The listing builds one solid part. Answer for the finished solid, in the listing's coordinates (mm). A direction names the side the tool comes from. Give positions to 0.01 mm unless a question says otherwise; leave off trailing zeros. Write each loop counter-clockwise with the first axis right and the second up, starting at its lowest first coordinate (ties: lowest second). Pieces come first, ordered by that corner, then holes. Notation, with made-up numbers: M 12,38.5 L 53,38.5 A19 cw 53,57.5 Z; hole C -17.5,-26.5 d11. An arc over 180 degrees is marked long. Return JSON: item names as keys, results as strings.
from build123d import *

# Parameters (mm, degrees)
POCKET002_DEPTH      = 20.001
POCKET002_DEPTH_BACK = -20.001
POCKET003_DEPTH      = 5
SKETCH004_R          = 5.2
POCKET004_DEPTH      = 26.045604
POCKET004_DEPTH_BACK = -21.981715
SKETCH007_R          = 15.2
SKETCH_R             = 20
SKETCH_R_2           = 15.3
PAD_DEPTH            = 9
SKETCH001_R          = 1.7
POCKET_DEPTH         = 134.561028
SKETCH002_R          = 2.95
POCKET001_DEPTH      = 2.5
SKETCH006_R          = 5.2
POCKET005_DEPTH      = 14.143136
POLARPATTERN_COUNT   = 3


with BuildPart() as body001:
    # Cone → Cone (revolve)
    with BuildSketch(Plane(origin=(0, 0, 9), x_dir=(1, 0, 0), z_dir=(0, -1, 0))):
        Polygon((0, 0), (20, 0), (0, 50), align=None)
    revolve(axis=Axis((0, 0, 9), (0, 0, 1)))

    # Sketch003 → Pocket002 (cut, two sides)
    with BuildSketch(Plane.YZ) as pocket002_sk:
        Polygon((22.25, 62.25), (-22.25, 17.75), (-27.75, 17.75), (-27.75, 67.75), (22.25, 67.75), align=None)
        Polygon((30.213203, 9), (-4.786797, 9), (-4.786797, 14), (30.213203, 49), align=None)
    extrude(amount=-POCKET002_DEPTH, mode=Mode.SUBTRACT)
    extrude(pocket002_sk.sketch, amount=-POCKET002_DEPTH_BACK, mode=Mode.SUBTRACT)

    # Sketch005 (on DatumPlane) → Pocket003 (cut)
    with BuildSketch(Plane(origin=(0, -0.79062, 33.552525), x_dir=(0, -0.707107, -0.707107), z_dir=(0, -0.707107, 0.707107))):
        Polygon((8.2, 0), (4.1, 7.101408), (-4.1, 7.101408), (-19.1, 7.101408), (-19.1, -7.101408), (-4.1, -7.101408), (4.1, -7.101408), align=None)
    extrude(amount=-POCKET003_DEPTH, mode=Mode.SUBTRACT)

    # Sketch004 (on DatumPlane) → Pocket004 (cut, two sides)
    with BuildSketch(Plane(origin=(0, -0.79062, 33.552525), x_dir=(0, -0.707107, -0.707107), z_dir=(0, -0.707107, 0.707107))) as pocket004_sk:
        Circle(SKETCH004_R)
    extrude(amount=-POCKET004_DEPTH, mode=Mode.SUBTRACT)
    extrude(pocket004_sk.sketch, amount=-POCKET004_DEPTH_BACK, mode=Mode.SUBTRACT)

    # SubtractivePipe: sweep along a path in Sketch008
    with BuildLine(Plane.YZ) as subtractivepipe_path:
        Line((0, 9), (28.284271, 37.284271))
    # Sketch007 (on Face1 of CopyPolarPattern) → SubtractivePipe (sweep, cut)
    with BuildSketch(Plane.XY.offset(9)):
        Circle(SKETCH007_R)
    sweep(path=subtractivepipe_path.line, mode=Mode.SUBTRACT)


with BuildPart() as body:
    # Sketch → Pad (new body)
    with BuildSketch(Plane.XY):
        Circle(SKETCH_R)
        Circle(SKETCH_R_2, mode=Mode.SUBTRACT)
    extrude(amount=PAD_DEPTH)

    # Sketch001 → Pocket (cut, through all)
    with BuildSketch(Plane.XZ):
        with Locations((0, 4.5)):
            Circle(SKETCH001_R)
    pocket = extrude(amount=POCKET_DEPTH, mode=Mode.SUBTRACT)

    # Sketch002 (on DatumPlane) → Pocket001 (cut)
    with BuildSketch(Plane.XZ.offset(20)):
        with Locations((0, 4.5)):
            Circle(SKETCH002_R)
    pocket001 = extrude(amount=-POCKET001_DEPTH, mode=Mode.SUBTRACT)

    # Sketch006 (on DatumPlane) → Pocket005 (cut, through all)
    with BuildSketch(Plane(origin=(0, 0, 0), x_dir=(1, 0, 0), z_dir=(0, -0.707107, 0.707107))):
        with Locations((0, 23.17)):
            Circle(SKETCH006_R)
    extrude(amount=-POCKET005_DEPTH, mode=Mode.SUBTRACT)

    # PolarPattern: Pocket, Pocket001 ×3 about axis
    polarpattern_axis = Axis((0, 0, 0), (0, 0, 1))
    for i in range(1, POLARPATTERN_COUNT):
        add(pocket.rotate(polarpattern_axis, i * 360 / POLARPATTERN_COUNT), mode=Mode.SUBTRACT)
        add(pocket001.rotate(polarpattern_axis, i * 360 / POLARPATTERN_COUNT), mode=Mode.SUBTRACT)

    # Boolean: union Body001
    add(body001.part)


solid = body.part
Item 1: Given pin 1 Ø1.8 at (x, z) = (1.5, 4) entering from -Y; pin 2 Ø10 at (x, z) = (-0.5, 26.5) entering from -Y; pin 3 Ø8.5 at (y, z) = (1.5, 32) entering from +X, each flat-ended and moving along its own axis, determine where each tip first touches the part or whether it passes through.
Geometry results:
{"pin 1": "stops at y = -17.5", "pin 2": "stops at y = -15", "pin 3": "stops at x = 12.45"}
Item 2: Which of the six approach directions +Z, -Z, +X, -X, +Y, -Y give full straight-line access (tool end or side, diameter ignored) to faces 1 (the cylindrical face through (-0.07, 18.179, 7.236)), 2 (the flat face through (3.256, 5.784, 33.056)), 3 (the flat face through (15, -4.787, 11))?
Geometry results:
{"face 1": "+Z, +Y", "face 2": "none", "face 3": "+X, -X, +Y"}
Item 3: A cutting plane is placed at A-A, the plane z = 4.5. Write down the section's boundary in (x, y).
Geometry results:
{"outline": "M -18.61,7.34 A20 ccw -2.95,-19.78 L -2.95,-17.5 L -1.7,-17.5 L -1.7,-15.21 A15.3 cw -14.02,6.13 L -16.01,7.28 L -16.63,6.2 Z; M -15.66,12.45 L -13.68,11.3 L -14.31,10.22 L -12.32,9.07 A15.3 cw 12.32,9.07 L 14.31,10.22 L 13.68,11.3 L 15.66,12.45 A20 ccw Z; M 1.7,-17.5 L 2.95,-17.5 L 2.95,-19.78 A20 ccw 18.61,7.34 L 16.63,6.2 L 16.01,7.28 L 14.02,6.13 A15.3 cw 1.7,-15.21 Z"}
Item 4: Find the intervals of material crossed by line 1 (Y direction, x = 0, z = 2); line 2 (X direction, y = 0, z = 2); line 3 (X direction, y = -2, z = 20), in increasing order.
Geometry results:
{"line 1": "y = -17.5 to -15.3, 15.3 to 20", "line 2": "x = -20 to -15.3, 15.3 to 20", "line 3": "x = -15.47 to -7.88, 7.88 to 15.47"}
Item 5: Determine the mould class of faces 4 (the cylindrical face through (-0.384, -18.768, 7.425)), 5 (the flat face through (-13.895, -0.407, 18.38)), 6 (the cylindrical face through (-4.336, -19.524, 4.437)) for opening direction X: +X half, -X half, draft (parallel to the pull), parting line (faces both ways), or undercut.
Geometry results:
{"face 4": "undercut", "face 5": "draft", "face 6": "parting line"}
